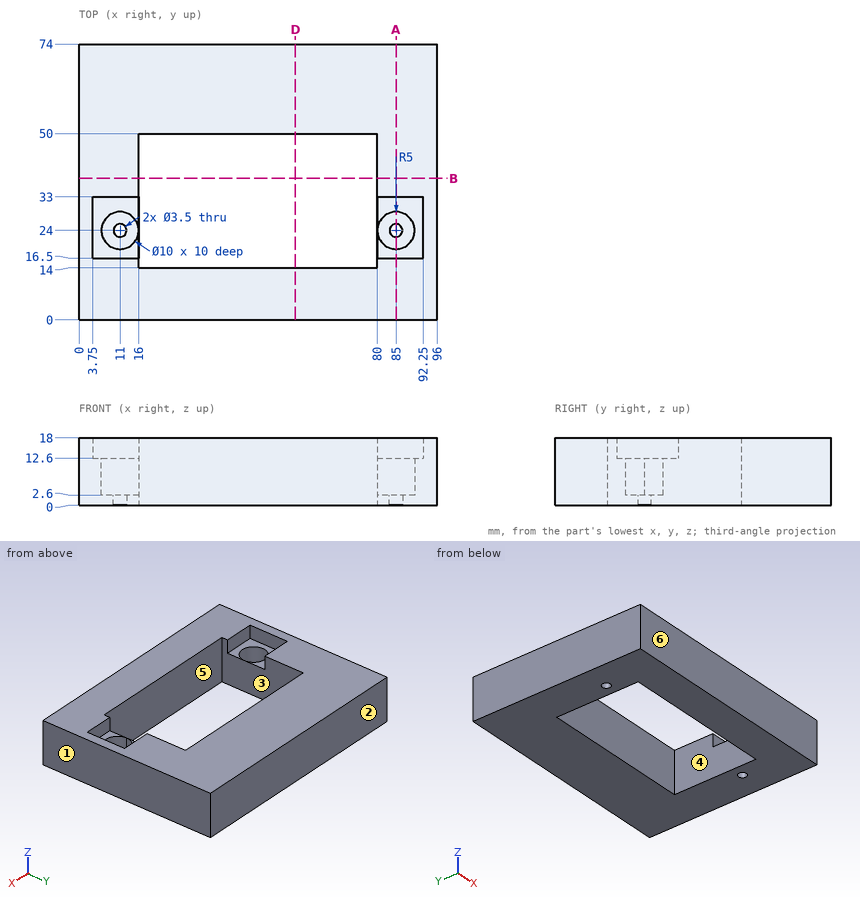
For this review, use the dimensioned drawing (mm, ordinates from the lowest corner) and the shaded views. A direction names the side the tool comes from. Round coordinates to 2 decimals unless told otherwise and drop trailing zeros. Write each loop counter-clockwise with the first axis right and the second up, starting at its lowest first coordinate (ties: lowest second). Pieces come first, ordered by that corner, then holes. Notation, with made-up numbers: (56, 12) -> (109, 12) arc R23 ccw to (109, 21) -> close; hole circle Ø5 at (-33, -38.5). An arc over 180 degrees is marked (long way). Use CSV: the item, a comma, the result in double quotes.
Q1. Consider section D-D (x = 58). Give the boundary of the cut face in (y, z), then the cut area to 3 significant figures.
Checks:
outline,"(0, 0) -> (14, 0) -> (14, 18) -> (0, 18) -> close; (50, 0) -> (74, 0) -> (74, 18) -> (50, 18) -> close"
area,"684 mm²"
Q2. For the marked faces 5 and 6, list the 3-axis set-ups (+Z, -Z, +X, -X, +Y, -Y) from which the entire face can be reached by the end or side of a thin tool; tool diameter is ignored.
Checks:
face 5,"+Z, -Z"
face 6,"+Z, -Z, +X, -X, -Y"
Q3. Mouldability with a two-part tool opening along X and no side actions: class the marked faces 1, 2, 3 and 4 as released by +X, released by -X, zero draft, split by the parting line, or undercut.
Checks:
face 1,"released by +X"
face 2,"zero draft"
face 3,"undercut"
face 4,"undercut"
Q4. Consider section B-B (y = 38). Give the boundary of the cut face in (x, z).
Checks:
outline,"(0, 0) -> (16, 0) -> (16, 18) -> (0, 18) -> close; (80, 0) -> (96, 0) -> (96, 18) -> (80, 18) -> close"
Q5. For pin 1 Ø2.5 at (y, z) = (26.5, 15) entering from -X; pin 2 Ø5 at (x, y) = (12, 22) entering from +Z; pin 3 Ø11.5 at (x, y) = (11, 24) entering from +Z, all flat-tipped, find the tip position at first contact; note any pin that passes through.
Checks:
pin 1,"x = 0"
pin 2,"z = 2.6"
pin 3,"z = 12.6"
Q6. To check wall thickness, follow probe 1 along X at (y, z) = (36.5, 3.5); probe 2 along Y at (x, z) = (74, 9.25); probe 3 along Y at (x, z) = (11, 0.75). State the ranges of each line that lie inside material, in increasing order. Write a range as [from, to].
Checks:
probe 1,"[0, 16], [80, 96]"
probe 2,"[0, 14], [50, 74]"
probe 3,"[0, 22.25], [25.75, 74]"
Q7. Consider section A-A (x = 85). Give the boundary of the cut face in (y, z).
Checks:
outline,"(0, 0) -> (22.25, 0) -> (22.25, 2.6) -> (19, 2.6) -> (19, 12.6) -> (16.5, 12.6) -> (16.5, 18) -> (0, 18) -> close; (25.75, 0) -> (74, 0) -> (74, 18) -> (33, 18) -> (33, 12.6) -> (29, 12.6) -> (29, 2.6) -> (25.75, 2.6) -> close"
